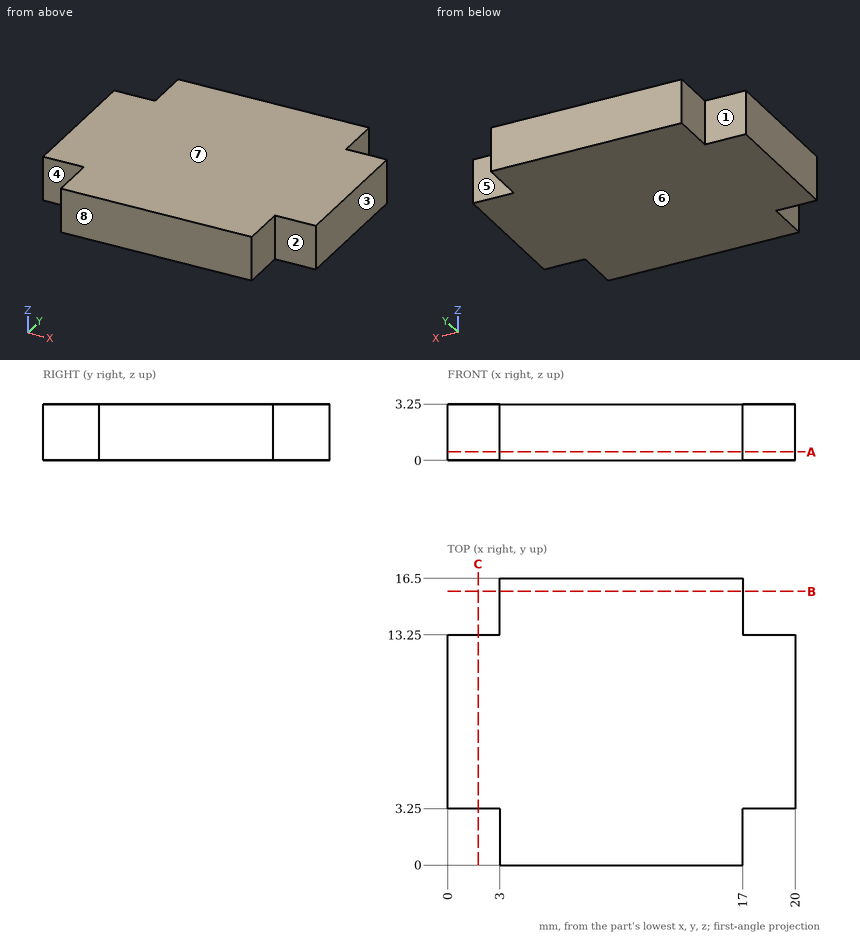
Can you work these out from the drawing? Everything is in mm from the part's minimum corner. A direction names the side the tool comes from. Round coordinates to 2 decimals unless told otherwise and drop trailing zeros. Write each loop counter-clockwise with the first axis right and the second up, starting at its lowest first coordinate (ties: lowest second). Pieces come first, ordered by that corner, then holes.
1. Suppose I cut it at C-C (x = 1.75). List the corners of the cut face in (y, z) for me, and give its area (3 significant figures).
2. Suppose I cut it at A-A (z = 0.5). List the corners of the cut face in (x, y) for me, and give its area (3 significant figures).
3. Suppose I cut it at B-B (y = 15.75). List the corners of the cut face in (x, z) for me, and give its area (3 significant figures).
4. If we mould it in two halves opening along Z, with no side actions, what happens to the marked faces 6, 7 and 8? For each: released by +Z, released by -Z, zero draft, split by the parting line, or undercut.
5. For the marked faces 1, 2, 3, 4 and 5, which set-ups out of +Z, -Z, +X, -X, +Y, -Y let a thin tool reach every point of the face, with its end or its side?
6. I need wall thicknesses on L1, parallel to Y at x = 18, z = 2.9; L2, parallel to X at y = 1.5, z = 0.85. Which ranges of each line are inside material? Lowest first, please.
7. Will these pins go through, and if not, where does the flat tip stop? pin 1 Ø1.6 at (y, z) = (15, 1) entering from -X; pin 2 Ø0.9 at (x, z) = (18.5, 1.5) entering from -Y; pin 3 Ø1.6 at (y, z) = (15, 2) entering from +X.
Answer sheet:
1. outline: (3.25, 0) - (13.25, 0) - (13.25, 3.25) - (3.25, 3.25) - close
1. area: 32.5 mm2
2. outline: (0, 3.25) - (3, 3.25) - (3, 0) - (17, 0) - (17, 3.25) - (20, 3.25) - (20, 13.25) - (17, 13.25) - (17, 16.5) - (3, 16.5) - (3, 13.25) - (0, 13.25) - close
2. area: 291 mm2
3. outline: (3, 0) - (17, 0) - (17, 3.25) - (3, 3.25) - close
3. area: 45.5 mm2
4. face 6: released by -Z
4. face 7: released by +Z
4. face 8: zero draft
5. face 1: +Z, -Z, -X, +Y
5. face 2: +Z, -Z, +X, -Y
5. face 3: +Z, -Z, +X, +Y, -Y
5. face 4: +Z, -Z, -X, -Y
5. face 5: +Z, -Z, +X, +Y
6. L1: y = 3.25 to 13.25
6. L2: x = 3 to 17
7. pin 1: stops at x = 3
7. pin 2: stops at y = 3.25
7. pin 3: stops at x = 17
